CAD build for the part. Positions are in the model's coordinates, mm. A direction names the side the tool comes from. Coordinates: 2 decimals unless noted, no trailing zeros. Loops run counter-clockwise (first coordinate to the right, second up) from the corner with the lowest first, then second, coordinate; pieces in that order, holes last. Notation, with made-up numbers: (12, -10) -> (47, -10) arc R34 cw to (47, 24) -> close; hole circle Ø6 at (84.25, 46). An arc over 180 degrees is marked (long way). Write item = value, one per line. Start each with the question number.
(1) Band-saw the part on B-B (y = -16). Write the cut outline in (x, z) (3 decimals).
(2) Drill centre lines: line 1 (X direction, y = -16.5, z = -4.25); line 2 (Y direction, x = -33.5, z = -4.5); line 3 (X direction, y = -61, z = 7). Where is each one in solid material? Low to high. Write a range as from..to.
(3) Band-saw the part on C-C (x = -14). Write the cut outline in (y, z) (3 decimals), and give its area (3 significant figures).
(4) Band-saw the part on A-A (x = -52.5). Write the cut outline in (y, z) (3 decimals), and give its area (3 significant figures).
(5) Flat gauge pins, fed straight in: P1, Ø4, axis at x = -61.5, y = -9, coming from the -Z side; P2, Ø1.5, axis at x = 12, y = -35, coming from the -Z side (3 decimals). Where does each tip first touch, or does it go through?
(6) Tool access for faces 1 (the face through (2, -72, 6.35)), 2 (the face through (-1, -12.7, -6)), 3 (the face through (-1, -144, -9.525)): list every direction of +Z, -Z, +X, -X, +Y, -Y with a clear straight run to the whole face (end or side of a thin tool).
(7) Band-saw the part on D-D (y = -50). Write the cut outline in (x, z) (3 decimals), and give its area (3 significant figures).
(8) Pull direction Y, two halves, no side cores. Call faces 4 (the face through (-57, -6, -9.366)), 5 (the face through (-3.438, -22.657, 7.96)), 6 (the face through (-1, -77, -3.175)), 7 (the face through (-2, 0, -1)): +Y half, -Y half, draft (parallel to the pull), parting line (faces both ways), or undercut.
```python
from build123d import *

# Parameters (mm, degrees)
F0_W     = 215.9
F0_H     = 19.05
F1_DEPTH = 152.4
F2_W     = 190.5
F2_H     = 127
F3_DEPTH = 6.35
F4_W     = 25.4
F4_H     = 12.7
F5_DEPTH = 0.15875
F6_R     = 3.175
F7_R     = 50.8
F8_DEPTH = 3.175


with BuildPart() as f1:
    # F0 (on Front) → F1 (new body)
    with BuildSketch(Plane.XZ):
        Rectangle(F0_W, F0_H)
    extrude(amount=F1_DEPTH)

    # F2 (on face) → F3 (cut)
    with BuildSketch(Plane(origin=(0, 0, -9.525), x_dir=(1, 0, 0), z_dir=(0, 0, -1))):
        with Locations((0, 76.2)):
            Rectangle(F2_W, F2_H)
    extrude(amount=-F3_DEPTH, mode=Mode.SUBTRACT)

    # F4 (on face) → F5 (cut)
    with BuildSketch(Plane(origin=(0, 0, -9.525), x_dir=(1, 0, 0), z_dir=(0, 0, -1))):
        with Locations((-57.15, 6.35)):
            Rectangle(F4_W, F4_H)
        with Locations((57.15, 6.35)):
            Rectangle(F4_W, F4_H)
    extrude(amount=-F5_DEPTH, mode=Mode.SUBTRACT)

    # F6
    f6_edges = [f1.edges().sort_by_distance(p)[0] for p in [
        (107.95, -76.2, 9.525),
        (-107.95, -76.2, 9.525),
        (0, 0, 9.525),
        (0, -152.4, 9.525),
    ]]
    fillet(f6_edges, radius=F6_R)

    # F7 (on face) → F8 (cut)
    with BuildSketch(Plane.XY.offset(9.525)):
        with Locations((3.175, -73.025)):
            Circle(F7_R)
    extrude(amount=-F8_DEPTH, mode=Mode.SUBTRACT)


solid = f1.part
```
Findings below:
q1.outline = (-107.95, -9.525) -> (-95.25, -9.525) -> (-95.25, -3.175) -> (95.25, -3.175) -> (95.25, -9.525) -> (107.95, -9.525) -> (107.95, 6.35) arc R3.175 ccw to (104.775, 9.525) -> (-104.775, 9.525) arc R3.175 ccw to (-107.95, 6.35) -> close
q2.line_1 = -107.95..-95.25, 95.25..107.95
q2.line_2 = -152.4..-139.7, -12.7..0
q2.line_3 = -107.88..-46.18, 52.53..107.88
q3.outline = (-152.4, -9.525) -> (-139.7, -9.525) -> (-139.7, -3.175) -> (-12.7, -3.175) -> (-12.7, -9.525) -> (0, -9.525) -> (0, 6.35) arc R3.175 ccw to (-3.175, 9.525) -> (-25.216, 9.525) -> (-25.216, 6.35) -> (-120.834, 6.35) -> (-120.834, 9.525) -> (-149.225, 9.525) arc R3.175 ccw to (-152.4, 6.35) -> close
q3.area = 1,790 mm²
q4.outline = (-152.4, -9.525) -> (-139.7, -9.525) -> (-139.7, -3.175) -> (-12.7, -3.175) -> (-12.7, -9.366) -> (0, -9.366) -> (0, 6.35) arc R3.175 ccw to (-3.175, 9.525) -> (-149.225, 9.525) arc R3.175 ccw to (-152.4, 6.35) -> close
q4.area = 2,090 mm²
q5.P1 = -9.37
q5.P2 = -3.175
q6.face_1 = +Z
q6.face_2 = -Z
q6.face_3 = -Z, +X, -X, +Y, -Y
q7.outline = (-107.95, -9.525) -> (-95.25, -9.525) -> (-95.25, -3.175) -> (95.25, -3.175) -> (95.25, -9.525) -> (107.95, -9.525) -> (107.95, 6.35) arc R3.175 ccw to (104.775, 9.525) -> (48.457, 9.525) -> (48.457, 6.35) -> (-42.107, 6.35) -> (-42.107, 9.525) -> (-104.775, 9.525) arc R3.175 ccw to (-107.95, 6.35) -> close
q7.area = 2,610 mm²
q8.face_4 = draft
q8.face_5 = undercut
q8.face_6 = undercut
q8.face_7 = +Y half
